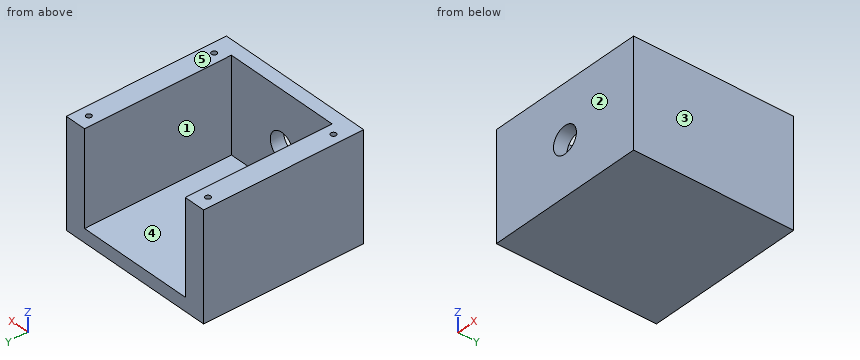
from build123d import *

# Parameters (mm, degrees)
F0_W     = 60
F0_H     = 40
F1_DEPTH = 60
F2_W     = 44
F2_H     = 55
F3_DEPTH = 35
F4_R     = 5
F5_DEPTH = 25
F7_R     = 1
F8_DEPTH = 5


with BuildPart() as f1:
    # F0 (on Front) → F1 (new body)
    with BuildSketch(Plane.XZ):
        Rectangle(F0_W, F0_H)
    extrude(amount=F1_DEPTH)

    # F2 (on face) → F3 (cut)
    with BuildSketch(Plane.XY.offset(20)):
        with Locations((0, -27.5)):
            Rectangle(F2_W, F2_H)
    extrude(amount=-F3_DEPTH, mode=Mode.SUBTRACT)

    # F4 (on face) → F5 (cut)
    with BuildSketch(Plane.XZ.offset(60)):
        Circle(F4_R)
    extrude(amount=-F5_DEPTH, mode=Mode.SUBTRACT)

    # F7 (on face) → F8 (cut)
    with BuildSketch(Plane.XY.offset(20)):
        with Locations((-26.1, -5)):
            Circle(F7_R)
        with Locations((26, -5)):
            Circle(F7_R)
        with Locations((26, -52)):
            Circle(F7_R)
        with Locations((-26.1, -52)):
            Circle(F7_R)
    extrude(amount=-F8_DEPTH, mode=Mode.SUBTRACT)


solid = f1.part
Geometry check sheet. Reference: the model listing, model coordinates, mm. Face numbers are marked on the shaded views. A direction names the side the tool comes from. Coordinates: 2 decimals unless noted, no trailing zeros. Order: outer loops, then holes, each group sorted by start corner. A loop starts at its lowest first (then second) coordinate and runs counter-clockwise, first axis right, second up. Notation, with made-up numbers: (57.25, 43) -> (115.25, 43) arc R10 cw to (115.25, 56) -> close; hole circle Ø9 at (30.5, 50.5). An arc over 180 degrees is marked (long way). Use a Markdown table: item, result. Add a question column.
1. Set-up check for the marked faces 1 and 2: record each of +Z, -Z, +X, -X, +Y, -Y from which the full face is reachable in a straight line by a thin tool's end or side.
2. Cross-section at B-B (z = -14). Enter the section's corners in (x, y), and give its area (3 significant figures).
3. Cross-section at C-C (y = -52). Enter the section's corners in (x, z).
4. Cross-section at D-D (z = 2). Enter the section's corners in (x, y).
5. Go/stop test with flat-tipped pins: pin 1 Ø6 at (x, z) = (13.5, -1) entering from +Y; pin 2 Ø1.8 at (x, y) = (26, -5) entering from +Z; pin 3 Ø12 at (x, y) = (8, -29) entering from +Z. Record where each tip stops, or that it passes through.
6. Material ranges on L1, parallel to Y at x = 26, z = 16; L2, parallel to X at y = -29.5, z = -8.5; L3, parallel to Z at x = -10, y = -54, recorded low to high.
7. Mould release check, pull along X, two halves, no side actions. Record for the marked faces 3, 4 and 5: pulls with the +X half, pulls with the -X half, needs draft (parallel to the pull), parting line crosses it, or undercut.
8. Cross-section at A-A (x = 0). Enter the section's corners in (y, z).
Filled sheet:
| question | item | result |
|---|---|---|
| 1 | face 1 | +Z, +Y |
| 1 | face 2 | +Z, -Z, +X, -X, -Y |
| 2 | outline | (-30, -60) -> (30, -60) -> (30, 0) -> (22, 0) -> (22, -55) -> (-22, -55) -> (-22, 0) -> (-30, 0) -> close |
| 2 | area | 1,180 mm2 |
| 3 | outline | (-30, -20) -> (30, -20) -> (30, 20) -> (27, 20) -> (27, 15) -> (25, 15) -> (25, 20) -> (22, 20) -> (22, -15) -> (-22, -15) -> (-22, 20) -> (-25.1, 20) -> (-25.1, 15) -> (-27.1, 15) -> (-27.1, 20) -> (-30, 20) -> close |
| 4 | outline | (-30, -60) -> (-4.58, -60) -> (-4.58, -55) -> (-22, -55) -> (-22, 0) -> (-30, 0) -> close; (4.58, -60) -> (30, -60) -> (30, 0) -> (22, 0) -> (22, -55) -> (4.58, -55) -> close |
| 5 | pin 1 | y = -55 |
| 5 | pin 2 | z = 15 |
| 5 | pin 3 | z = -15 |
| 6 | L1 | -60 to -53, -51 to -6, -4 to 0 |
| 6 | L2 | -30 to -22, 22 to 30 |
| 6 | L3 | -20 to -15 |
| 7 | face 3 | pulls with the +X half |
| 7 | face 4 | undercut |
| 7 | face 5 | needs draft |
| 8 | outline | (-60, -20) -> (0, -20) -> (0, -15) -> (-55, -15) -> (-55, -5) -> (-60, -5) -> close; (-60, 5) -> (-55, 5) -> (-55, 20) -> (-60, 20) -> close |
